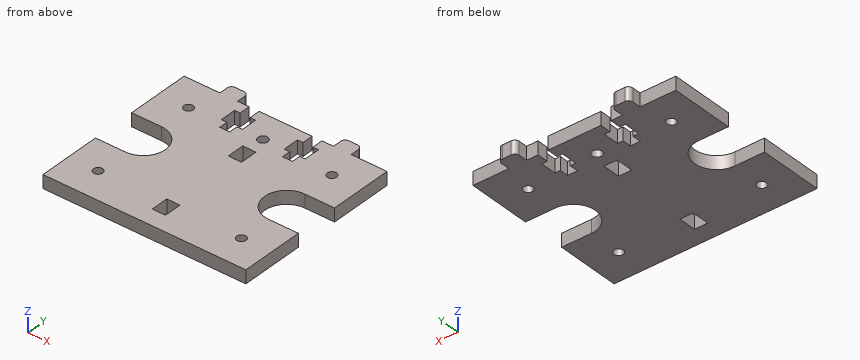
Autodesk Inventor part; units mm, degrees
ref_plane "YZ Plane" through (0, 0, 0) normal (1, 0, 0) x (0, 1, 0)
ref_plane "XZ Plane" through (0, 0, 0) normal (0, 1, 0) x (-1, 0, 0)
ref_plane "XY Plane" through (0, 0, 0) normal (0, 0, 1) x (1, 0, 0)
sketch "Sketch1" plane through (0, 0, 0) normal (0, 0, 1) x (1, 0, 0)
  line L0 (0, 0) -> (92, 0)
  line L1 (92, 78) -> (0, 78)
  line L2 (0, 49) -> (13.5, 49)
  arc A0 (13.5, 29) -> (13.5, 49) centre (13.5, 39) ccw
  line L3 (13.5, 29) -> (0, 29)
  line L4 (92, 49) -> (78.5, 49)
  arc A1 (78.5, 49) -> (78.5, 29) centre (78.5, 39) ccw
  line L5 (78.5, 29) -> (92, 29)
  line L6 (0, 78) -> (0, 49)
  line L7 (0, 29) -> (0, 0)
  line L8 (92, 0) -> (92, 29)
  line L9 (92, 49) -> (92, 78)
  dimension "d0" = 92
  dimension "d1" = 20
  dimension "d2" = 78
  dimension "d3" = 39
  dimension "d11" = 65
extrude "Extrusion1" add sketch "Sketch1" along normal blind 6
sketch "Sketch2" plane through (0, 0, 6) normal (0, 0, 1) x (1, 0, 0)
  arc A0 (78.5, 49) -> (78.5, 29) centre (78.5, 39) ccw
  arc A1 (13.5, 29) -> (13.5, 49) centre (13.5, 39) ccw
  line L0 (13.5, 64) -> (78.5, 64) construction
  line L1 (78.5, 64) -> (78.5, 14) construction
  line L2 (78.5, 14) -> (13.5, 14) construction
  line L3 (13.5, 14) -> (13.5, 64) construction
  circle A2 centre (13.5, 64) radius 2.1
  circle A3 centre (13.5, 14) radius 2.1
  circle A4 centre (78.5, 14) radius 2.1
  circle A5 centre (78.5, 64) radius 2.1
  dimension "d7" = 4.2
  dimension "d8" = 50
extrude "Extrusion2" cut sketch "Sketch2" against normal blind 6
sketch "Sketch3" plane through (0, 0, 6) normal (0, 0, 1) x (1, 0, 0)
  line L0 (92, 78) -> (0, 78)
  line L1 (29.5, 78) -> (34, 78)
  line L2 (34, 61.7) -> (29.5, 61.7)
  line L3 (36.5, 73) -> (36.5, 65.7)
  line L4 (27, 65.7) -> (27, 73)
  line L5 (34, 78) -> (34, 73)
  line L6 (34, 65.7) -> (34, 61.7)
  line L7 (29.5, 61.7) -> (29.5, 65.7)
  line L8 (29.5, 73) -> (29.5, 78)
  line L9 (27, 73) -> (29.5, 73)
  line L10 (34, 73) -> (36.5, 73)
  line L11 (36.5, 65.7) -> (34, 65.7)
  line L12 (29.5, 65.7) -> (27, 65.7)
  line L13 (58, 78) -> (62.5, 78)
  line L14 (62.5, 61.7) -> (58, 61.7)
  line L15 (65, 73) -> (65, 65.7)
  line L16 (55.5, 65.7) -> (55.5, 73)
  line L17 (62.5, 78) -> (62.5, 73)
  line L18 (62.5, 65.7) -> (62.5, 61.7)
  line L19 (58, 61.7) -> (58, 65.7)
  line L20 (58, 73) -> (58, 78)
  line L21 (55.5, 73) -> (58, 73)
  line L22 (62.5, 73) -> (65, 73)
  line L23 (65, 65.7) -> (62.5, 65.7)
  line L24 (58, 65.7) -> (55.5, 65.7)
  line L25 (36.5, 69.35) -> (55.5, 69.35) construction
  point P0 (31.75, 61.7)
  point P1 (60.25, 61.7)
  point P2 (46, 69.35)
  point P3 (46, 78)
  dimension "d12" = 7.3
  dimension "d13" = 4
  dimension "d14" = 5
  dimension "d15" = 2.5
  dimension "d16" = 4.5
  dimension "d17" = 7.3
  dimension "d18" = 4
  dimension "d19" = 5
  dimension "d20" = 2.5
  dimension "d21" = 4.5
  dimension "d22" = 38
extrude "Extrusion3" cut sketch "Sketch3" against normal blind 6
sketch "Sketch4" plane through (0, 0, 6) normal (0, 0, 1) x (1, 0, 0)
  line L0 (29.5, 78) -> (0, 78)
  line L1 (92, 78) -> (62.5, 78)
  line L2 (62.5, 61.7) -> (58, 61.7)
  line L3 (34, 61.7) -> (29.5, 61.7)
  line L4 (16.25, 78) -> (24.25, 78)
  line L5 (24.25, 78) -> (24.25, 82)
  line L6 (22.25, 84) -> (18.25, 84)
  line L7 (16.25, 82) -> (16.25, 78)
  line L8 (67.75, 78) -> (75.75, 78)
  line L9 (75.75, 78) -> (75.75, 82)
  line L10 (73.75, 84) -> (69.75, 84)
  line L11 (67.75, 82) -> (67.75, 78)
  arc A0 (18.25, 84) -> (16.25, 82) centre (18.25, 82) ccw
  arc A1 (24.25, 82) -> (22.25, 84) centre (22.25, 82) ccw
  arc A2 (69.75, 84) -> (67.75, 82) centre (69.75, 82) ccw
  arc A3 (75.75, 82) -> (73.75, 84) centre (73.75, 82) ccw
  point P0 (31.75, 61.7)
  point P1 (60.25, 61.7)
  dimension "d25" = 2
  dimension "d26" = 8
  dimension "d27" = 8
  dimension "d28" = 7.5
  dimension "d29" = 7.5
  dimension "d30" = 6
extrude "Extrusion4" add sketch "Sketch4" against normal blind 6
sketch "Sketch5" plane through (0, 0, 6) normal (0, 0, 1) x (1, 0, 0)
  line L0 (0, 0) -> (92, 0)
  line L1 (58, 78) -> (34, 78)
  line L2 (43, 58) -> (49, 58)
  line L3 (49, 58) -> (49, 50)
  line L4 (49, 50) -> (43, 50)
  line L5 (43, 50) -> (43, 58)
  line L6 (43, 16) -> (49, 16)
  line L7 (49, 16) -> (49, 8)
  line L8 (49, 8) -> (43, 8)
  line L9 (43, 8) -> (43, 16)
  point P0 (46, 0)
  point P1 (46, 8)
  dimension "d33" = 6
  dimension "d34" = 8
  dimension "d35" = 20
  dimension "d36" = 8
extrude "Extrusion5" cut sketch "Sketch5" against normal blind 6
sketch "Sketch6" plane through (0, 0, 6) normal (0, 0, 1) x (1, 0, 0)
  line L0 (43, 58) -> (49, 58)
  line L1 (58, 78) -> (34, 78)
  circle A0 centre (46, 65.5) radius 2.25
  point P0 (46, 58)
  dimension "d39" = 4.5
  dimension "d40" = 12.5
extrude "Extrusion6" cut sketch "Sketch6" against normal through all
equation "\"d3\" = 0.5 * d2"
properties part number "x_carryage_extruder_mount"
Check sheet for the modelled part. Datum: model origin and axes. Units: mm. Coordinates: 2 decimals unless noted, no trailing zeros. Write each loop counter-clockwise with the first axis right and the second up, starting at its lowest first coordinate (ties: lowest second). Pieces come first, ordered by that corner, then holes. Notation, with made-up numbers: (76, 2.25) -> (120, 2.25) arc R27 cw to (120, 18.25) -> close; hole circle Ø9 at (86.25, -12). An arc over 180 degrees is marked (long way). Use a Markdown table: item, result.
1. Sectioned sample at A-A (x = 64). Enter the section's corners in (y, z), plus the area to 3 significant figures.
Reported:
| item | result |
|---|---|
| outline | (0, 0) -> (65.7, 0) -> (65.7, 6) -> (0, 6) -> close; (73, 0) -> (78, 0) -> (78, 6) -> (73, 6) -> close |
| area | 424 mm2 |
2. Scan lines: line 1 along Y through (x, z) = (78.5, 3.15); line 2 along Y through (x, z) = (82, 4.3); line 3 along Y through (x, z) = (12, 3.75). Record each from-to range of solid material in increasing order.
Reported:
| item | result |
|---|---|
| line 1 | y = 0 to 11.9, 16.1 to 29, 49 to 61.9, 66.1 to 78 |
| line 2 | y = 0 to 29, 49 to 78 |
| line 3 | y = 0 to 12.53, 15.47 to 29, 49 to 62.53, 65.47 to 78 |
3. Go/stop test with flat-tipped pins: pin 1 Ø3 at (y, z) = (13, 3) entering from -X; pin 2 Ø0.8 at (x, z) = (35, 2.5) entering from +Y; pin 3 Ø2 at (y, z) = (79.5, 2.5) entering from +X; pin 4 Ø2 at (x, z) = (60, 1.5) entering from +Y. Record where each tip stops, or that it passes through.
Reported:
| item | result |
|---|---|
| pin 1 | stops at x = 0 |
| pin 2 | stops at y = 78 |
| pin 3 | stops at x = 75.75 |
| pin 4 | stops at y = 61.7 |
4. Sectioned sample at C-C (z = 1.1). Give the number of separate pieces and of enclosed holes in the cut face, plus the area to 3 significant figures.
Reported:
| item | result |
|---|---|
| separate pieces | 1 |
| enclosed holes | 7 |
| area | 6,030 mm2 |
5. Sectioned sample at D-D (y = 39). Enter the section's corners in (x, z), plus the area to 3 significant figures.
Reported:
| item | result |
|---|---|
| outline | (23.5, 0) -> (68.5, 0) -> (68.5, 6) -> (23.5, 6) -> close |
| area | 270 mm2 |
6. Sectioned sample at B-B (y = 14). Enter the section's corners in (x, z).
Reported:
| item | result |
|---|---|
| outline | (0, 0) -> (11.4, 0) -> (11.4, 6) -> (0, 6) -> close; (15.6, 0) -> (43, 0) -> (43, 6) -> (15.6, 6) -> close; (49, 0) -> (76.4, 0) -> (76.4, 6) -> (49, 6) -> close; (80.6, 0) -> (92, 0) -> (92, 6) -> (80.6, 6) -> close |
